Check sheet for the modelled part. Datum: model origin and axes. Units: mm. Give positions to 0.01 mm unless a question says otherwise; leave off trailing zeros. Order: outer loops, then holes, each group sorted by start corner. A loop starts at its lowest first (then second) coordinate and runs counter-clockwise, first axis right, second up. Notation, with made-up numbers: (58, 27.25) -> (85, 27.25) arc R29 ccw to (85, 48.25) -> close; hole circle Ø8 at (-28, -7.5). An arc over 180 degrees is marked (long way). Write each question's results on one line, items separated by ' | '.
Autodesk Inventor part; units mm, degrees
ref_plane "YZ Plane" through (0, 0, 0) normal (1, 0, 0) x (0, 1, 0)
ref_plane "XZ Plane" through (0, 0, 0) normal (0, 1, 0) x (-1, 0, 0)
ref_plane "XY Plane" through (0, 0, 0) normal (0, 0, 1) x (1, 0, 0)
sketch "草图1" plane through (0, 0, 0) normal (0, 0, 1) x (1, 0, 0)
  line L0 (-326.5872, 86.4864) -> (428.4128, 86.4864)
  line L1 (428.4128, 86.4864) -> (428.4128, 71.4864)
  line L2 (-326.5872, 71.4864) -> (-326.5872, 86.4864)
  line L3 (428.4128, 11.4864) -> (428.4128, -3.5136)
  line L4 (428.4128, -3.5136) -> (-326.5872, -3.5136)
  line L5 (-326.5872, -3.5136) -> (-326.5872, 11.4864)
  line L6 (-284.5872, 71.4864) -> (-284.5872, 11.4864)
  line L7 (-296.5872, 11.4864) -> (-296.5872, 71.4864)
  line L8 (398.4128, 71.4864) -> (398.4128, 11.4864)
  line L9 (386.4128, 11.4864) -> (386.4128, 71.4864)
  line L10 (-296.5872, 71.4864) -> (-326.5872, 71.4864)
  line L11 (-326.5872, 11.4864) -> (-296.5872, 11.4864)
  line L12 (428.4128, 71.4864) -> (398.4128, 71.4864)
  line L13 (386.4128, 71.4864) -> (-284.5872, 71.4864)
  line L14 (-284.5872, 11.4864) -> (386.4128, 11.4864)
  line L15 (398.4128, 11.4864) -> (428.4128, 11.4864)
  point P0 (0, 0)
  point P1 (-326.5872, 78.9864)
  point P2 (-326.5872, 3.9864)
  dimension "d0" = 755
  dimension "d1" = 15
  dimension "d2" = 15
  dimension "d3" = 7.5
  dimension "d4" = 75
  dimension "d5" = 12
  dimension "d6" = 12
  dimension "d7" = 30
  dimension "d8" = 30
extrude "拉伸1" add sketch "草图1" along normal blind 15
fillet "圆角1" radius 5 1 edges at (50.9128, 86.4864, 15)
fillet "圆角2" radius 5 12 edges at (50.9128, 86.4864, 0) (50.9128, 71.4864, 15) (413.4128, 71.4864, 15) (413.4128, 11.4864, 15) (413.4128, 11.4864, 0) (50.9128, -3.5136, 15) (50.9128, 11.4864, 15) (50.9128, 11.4864, 0) (50.9128, -3.5136, 0) (-311.5872, 11.4864, 15) (-311.5872, 71.4864, 15) (-311.5872, 71.4864, 0)
fillet "圆角3" radius 5 3 edges at (-311.5872, 11.4864, 0) (413.4128, 71.4864, 0) (50.9128, 71.4864, 0)
sketch "草图2" plane through (428.4128, 76.4864, 15) normal (1, 0, 0) x (0, 0, -1)
  line L0 (15, 5) -> (15, 0)
  line L1 (10, -5) -> (5, -5)
  circle A0 centre (7.5, 2.5) radius 2.5
  circle A1 centre (7.5, -72.5) radius 2.5
  line L2 (15, -70) -> (15, -75)
  line L3 (10, -65) -> (5, -65)
  point P0 (15, -76.4864)
  dimension "d14" = 7.5
  dimension "d15" = 7.5
  dimension "d16" = 7.5
  dimension "d17" = 7.5
  dimension "d18" = 5
extrude "拉伸2" cut sketch "草图2" against normal blind 800
properties part number "Desk foot holding bar"
1. Section check C-C on x = 256. Record the cut outline in (y, z).
Verdict:
outline: (-3.51, 5) arc R5 ccw to (1.49, 0) -> (6.49, 0) arc R5 ccw to (11.49, 5) -> (11.49, 10) arc R5 ccw to (6.49, 15) -> (1.49, 15) arc R5 ccw to (-3.51, 10) -> close; (71.49, 5) arc R5 ccw to (76.49, 0) -> (81.49, 0) arc R5 ccw to (86.49, 5) -> (86.49, 10) arc R5 ccw to (81.49, 15) -> (76.49, 15) arc R5 ccw to (71.49, 10) -> close; hole circle Ø5 at (3.99, 7.5); hole circle Ø5 at (78.99, 7.5)
2. Mould release check, pull along X, two halves, no side actions. Record for faces 1 (the flat face through (386.413, 41, 7)), 2 (the flat face through (-7, 6, 15)), 3 (the flat face through (-326.587, 79, 11)), 4 (the flat face through (398.413, 42, 7)): +X half, -X half, draft (parallel to the pull), parting line (faces both ways), or undercut.
Verdict:
face 1: undercut | face 2: draft | face 3: -X half | face 4: +X half
3. Section check B-B on y = 48. Record the cut outline in (x, z).
Verdict:
outline: (-296.59, 0) -> (-284.59, 0) -> (-284.59, 15) -> (-296.59, 15) -> close; (386.41, 0) -> (398.41, 0) -> (398.41, 15) -> (386.41, 15) -> close
4. Gauge pin test, flat ends, axial feed: pin 1 Ø7.5 at (y, z) = (28.5, 11) entering from +X; pin 2 Ø8 at (y, z) = (70, 3.5) entering from +X; pin 3 Ø1 at (y, z) = (49, 4) entering from -X; pin 4 Ø12 at (x, y) = (59, 69) entering from +Z. Record the tip position at first contact, or that the pin passes through.
Verdict:
pin 1: stops at x = 398.41 | pin 2: stops at x = 428.41 | pin 3: stops at x = -296.59 | pin 4: stops at z = 14.77
5. Section check A-A on z = 7.5. Record the cut outline in (x, y), then the cut area to 3 significant figures.
Verdict:
outline: (-326.59, -3.51) -> (428.41, -3.51) -> (428.41, 1.49) -> (-326.59, 1.49) -> close; (-326.59, 6.49) -> (428.41, 6.49) -> (428.41, 11.49) -> (398.41, 11.49) -> (398.41, 71.49) -> (428.41, 71.49) -> (428.41, 76.49) -> (-326.59, 76.49) -> (-326.59, 71.49) -> (-296.59, 71.49) -> (-296.59, 11.49) -> (-326.59, 11.49) -> close; (-326.59, 81.49) -> (428.41, 81.49) -> (428.41, 86.49) -> (-326.59, 86.49) -> close; hole (-284.59, 11.49) -> (386.41, 11.49) -> (386.41, 71.49) -> (-284.59, 71.49) -> close | area: 16,500 mm^2
6. Material ranges on probe 1 along Y at (x, z) = (-83.5, 7.5); probe 2 along X at (y, z) = (46.5, 12.5); probe 3 along Y at (x, z) = (-146.5, 5.5), recorded low to high. Write a range as from..to.
Verdict:
probe 1: y = -3.51..1.49, 6.49..11.49, 71.49..76.49, 81.49..86.49 | probe 2: x = -296.59..-284.59, 386.41..398.41 | probe 3: y = -3.51..2.49, 5.49..11.49, 71.49..77.49, 80.49..86.49
